Model file for the job. Use its own axes, mm. A direction names the side the tool comes from. Give positions to 0.01 mm unless a question says otherwise; leave off trailing zeros. Loops run counter-clockwise (first coordinate to the right, second up) from the corner with the lowest first, then second, coordinate; pieces in that order, holes last. Notation, with made-up numbers: M 19.25,88 L 40.25,88 A28 cw 40.25,117 Z; hole C -24.5,47 d1. An arc over 180 degrees is marked long. Answer in a Markdown table with one row per item.
Autodesk Inventor part; units mm, degrees
ref_plane "Work Plane1" through (-25.4, 0, 31.75) normal (0, 0, 1) x (1, 0, 0)
ref_plane "YZ Plane" through (0, 0, 0) normal (1, 0, 0) x (0, 1, 0)
ref_plane "XZ Plane" through (0, 0, 0) normal (0, 1, 0) x (-1, 0, 0)
sketch "Sketch1" plane through (0, 0, 0) normal (0, 1, 0) x (-1, 0, 0)
  line L0 (-25.4, 57.15) -> (25.4, 57.15)
  line L1 (25.4, 57.15) -> (25.4, -57.15)
  line L2 (25.4, -57.15) -> (-25.4, -57.15)
  line L3 (-25.4, -57.15) -> (-25.4, 57.15)
  line L4 (-25.4, 57.15) -> (25.4, -57.15) construction
  line L5 (25.4, 57.15) -> (-25.4, -57.15) construction
  point P0 (0, 0)
  dimension "d0" = 50.8
  dimension "d1" = 114.3
extrude "Extrusion1" add sketch "Sketch1" along normal blind 15.875
ref_plane "Work Plane1" through (-25.4, 0, 31.75) normal (0, 0, 1) x (1, 0, 0)
sketch "Sketch2" plane through (-25.4, 0, 31.75) normal (0, 0, 1) x (1, 0, 0)
  line L0 (50.8, 0) -> (0, 0) construction
  line L1 (50.8, 0) -> (50.8, 15.875) construction
  line L2 (0, 15.875) -> (50.8, 15.875) construction
  line L3 (0, 0) -> (0, 15.875) construction
  line L4 (0, 15.875) -> (50.8, 15.875) construction
  line L5 (25.4, 15.875) -> (25.4, 0) construction
  line L6 (50.8, 0) -> (0, 0) construction
  line L7 (6.35, 15.875) -> (6.35, 0) construction
  circle A0 centre (25.4, 16.891) radius 5.08 construction
  line L8 (12.7, 15.875) -> (12.7, 12.7)
  line L9 (12.7, 12.7) -> (9.525, 10.8669)
  line L10 (9.525, 10.8669) -> (9.525, 7.9375)
  line L11 (9.525, 7.9375) -> (19.05, 7.9375)
  line L12 (19.05, 7.9375) -> (19.05, 3.175)
  line L13 (19.05, 3.175) -> (25.4, 3.175)
  line L14 (12.7, 15.875) -> (25.4, 15.875)
  line L15 (25.4, 15.875) -> (25.4, 3.175)
  line L16 (19.05, 7.9375) -> (25.4, 7.9375)
  line L17 (20.6375, 7.9375) -> (20.6375, 7.2665)
  line L18 (20.6375, 7.2665) -> (22.225, 6.35)
  line L19 (22.225, 6.35) -> (22.225, 3.175)
  point P0 (22.225, 4.7625)
  point P1 (19.05, 5.5562)
  dimension "d20" = 6.35
  dimension "d21" = 10.16
  dimension "d22" = 6.35
  dimension "d23" = 4.7625
  dimension "d24" = 3.175
  dimension "d25" = 3.175
  dimension "d26" = 30
  dimension "d27" = 3.175
  dimension "d28" = 3.175
  dimension "d29" = 1.016
  dimension "d45" = 1.5875
  dimension "d46" = 3.175
  dimension "d48" = 3.175
  dimension "d50" = 30
extrude "Extrusion2" cut sketch "Sketch2" against normal through all
extrude "Extrusion3" cut sketch "Sketch2" along normal through all contours L14 L15 L16 L11 L10 L9 L8 | L17 L18 L19 L13 L12 L16
sketch "Sketch7" plane through (-6.35, 3.175, -57.15) normal (0, 1, 0) x (1, 0, 0)
  line L0 (0, -114.3) -> (0, 0) construction
  line L1 (6.35, -114.3) -> (1.5875, -114.3) construction
  line L2 (6.35, -88.9) -> (6.35, -114.3) construction
  line L3 (1.5875, -88.9) -> (6.35, -88.9) construction
  line L4 (1.5875, -88.9) -> (1.5875, -114.3) construction
  line L5 (0, -87.63) -> (1.5875, -86.0425)
  line L6 (1.5875, -86.0425) -> (1.5875, 0)
  line L7 (-19.05, 0) -> (31.75, 0)
  line L8 (0, 0) -> (1.5875, 0)
  line L9 (0, 0) -> (0, -87.63)
  point P0 (6.35, -57.15)
  dimension "d63" = 135
  dimension "d64" = 1.5875
  dimension "d65" = 1.27
extrude "Extrusion6" add sketch "Sketch7" along normal up to surface (4.7625 mm away)
chamfer "Chamfer2" distance 0.762 angle 45 2 edges at (-4.7625, 7.602, 31.75) (-3.175, 4.7625, 57.15)
sketch "Sketch8" plane through (0, 15.875, 0) normal (0, 1, 0) x (1, 0, 0)
  circle A0 centre (-20.32, 26.67) radius 2.5797 construction
  line L0 (-12.7, 57.15) -> (-25.4, 57.15) construction
  line L1 (-25.4, 57.15) -> (-25.4, -57.15) construction
  line L2 (-15.875, -57.15) -> (-15.875, 57.15) construction
  line L3 (-25.4, -57.15) -> (25.4, -57.15)
  line L4 (-25.4, 22.86) -> (-19.05, 16.51)
  line L5 (-19.05, 16.51) -> (-19.05, -41.91)
  line L6 (-19.05, -41.91) -> (-25.4, -48.26)
  line L7 (-25.4, 22.86) -> (-25.4, -48.26)
  line L8 (-25.4, -57.15) -> (-25.4, 57.15) construction
  line L9 (-25.4, 30.48) -> (-19.05, 36.83)
  line L10 (-19.05, 36.83) -> (-19.05, 57.15)
  line L11 (-25.4, 30.48) -> (-25.4, 22.86) construction
  line L12 (-25.4, 30.48) -> (-25.4, 57.15)
  line L13 (-25.4, 57.15) -> (-19.05, 57.15)
  point P0 (0, 0)
  point P1 (-20.32, -52.07)
  point P2 (-12.7, -57.15)
  point P3 (-25.4, 26.67)
  dimension "d71" = 5.1594
  dimension "d72" = 30.48
  dimension "d73" = 5.08
  dimension "d75" = 135
  dimension "d76" = 135
  dimension "d77" = 3.175
  dimension "d89" = 34.29
  dimension "d91" = 5.08
  dimension "d92" = 8.89
hole "Hole2" at (-20.32, 15.875, -26.67) at (-20.32, 15.875, 52.07) direction (0, -1, 0) diameter 5.1562 end through all
extrude "Extrusion7" cut sketch "Sketch8" against normal through all
mirror "Mirror1" about plane through (0, 15.875, 31.75) normal (-1, 0, 0) of "Extrusion2", "Extrusion3", "Extrusion7", "Hole2", "Chamfer2", "Extrusion6"
sketch "Sketch9" plane through (0, 0, 0) normal (0, -1, 0) x (1, 0, 0)
  line L0 (19.05, -57.15) -> (19.05, -36.83)
  line L1 (19.05, -57.15) -> (12.7, -57.15)
  line L2 (-19.05, -57.15) -> (-19.05, -36.83)
  line L3 (19.05, -57.15) -> (-19.05, -57.15)
  line L4 (-19.05, -57.15) -> (-19.05, -40.64)
  line L5 (-19.05, -40.64) -> (19.05, -40.64)
  line L6 (19.05, -40.64) -> (19.05, -57.15)
  point P0 (0, 0)
  dimension "d93" = 16.51
extrude "Extrusion8" cut sketch "Sketch9" against normal through all
equation "\"d76\" = d75"
properties part number "Holder_Mount" material "ABS Plastic"
Q1. Saw through at C-C (y = 1.75). Give the cut face in (x, z), and give its area (3 significant figures).
Reported:
| item | result |
|---|---|
| outline | M -25.4,-30.48 L -19.05,-36.83 L -19.05,-40.64 L 19.05,-40.64 L 19.05,-36.83 L 25.4,-30.48 L 25.4,-22.86 L 19.05,-16.51 L 19.05,41.91 L 25.4,48.26 L 25.4,57.15 L -25.4,57.15 L -25.4,48.26 L -19.05,41.91 L -19.05,-16.51 L -25.4,-22.86 Z; hole C -20.32,-26.67 d5.16; hole C -20.32,52.07 d5.16; hole C 20.32,-26.67 d5.16; hole C 20.32,52.07 d5.16 |
| area | 3,970 mm² |
Q2. Saw through at B-B (x = -20.32). Give the cut face in (y, z) (3 decimals), and give its area (3 significant figures).
Reported:
| item | result |
|---|---|
| outline | M 0,-35.56 L 15.875,-35.56 L 15.875,-29.248 L 0,-29.248 Z; M 0,-24.092 L 15.875,-24.092 L 15.875,-17.78 L 0,-17.78 Z; M 0,43.18 L 15.875,43.18 L 15.875,49.492 L 0,49.492 Z; M 0,54.648 L 15.875,54.648 L 15.875,57.15 L 0,57.15 Z |
| area | 340 mm² |
Q3. 3-axis set-ups, long thin cutter, end or side, ignore diameter. For faces 4 (the face through (-15.875, 9, 8)), 5 (the face through (-19.05, 8, -39)), 6 (the face through (-22.27, 8.05, -19.73)): which of +Z, -Z, +X, -X, +Y, -Y reach the whole face in a straight line?
Reported:
| item | result |
|---|---|
| face 4 | +Z, -Z |
| face 5 | -Z, -X, +Y, -Y |
| face 6 | -X, +Y, -Y |
Q4. Saw through at A-A (z = -26.67). Give the cut face in (x, y) (1 decimal).
Reported:
| item | result |
|---|---|
| outline | M -25.4,0 L -22.9,0 L -22.9,15.9 L -25.4,15.9 Z; M -17.7,0 L 17.7,0 L 17.7,15.9 L 12.7,15.9 L 12.7,12.7 L 15.9,10.9 L 15.9,7.9 L 4.8,7.9 L 4.8,3.2 L -4.8,3.2 L -4.8,7.9 L -15.9,7.9 L -15.9,10.9 L -12.7,12.7 L -12.7,15.9 L -17.7,15.9 Z; M 22.9,0 L 25.4,0 L 25.4,15.9 L 22.9,15.9 Z |
Q5. Probe probe 1 along X at (y, z) = (3.5, -26.67); probe 2 along X at (y, z) = (7.75, 34); probe 3 along X at (y, z) = (5.5, 52.07) (3 decimals). List the from-to ranges inside material, lowest first.
Reported:
| item | result |
|---|---|
| probe 1 | -25.4 to -22.9, -17.74 to -4.76, 4.76 to 17.74, 22.9 to 25.4 |
| probe 2 | -19.05 to -6.35, -4.76 to 4.76, 6.35 to 19.05 |
| probe 3 | -25.4 to -22.898, -17.742 to -6.35, -3.175 to 3.175, 6.35 to 17.742, 22.898 to 25.4 |
Q6. Drop flat-ended pins along their axis: pin 1 (2.5 mm diameter, centred on y = 4.5, z = 38.5, fed in from +X); pin 2 (5 mm diameter, centred on x = 2, z = 46.5, fed in from +Y); pin 3 (3 mm diameter, centred on y = 9.5, z = -38.5, fed in from -X). Give the stop position or say it passes through.
Reported:
| item | result |
|---|---|
| pin 1 | x = 19.05 |
| pin 2 | y = 7.94 |
| pin 3 | x = -19.05 |
Q7. Mould opens along Z. For faces 1 (the face through (-17.803, 7.826, 51.511)), 2 (the face through (4.09, 6.88, 44.27)), 3 (the face through (0, 6, 31.75)) say: released by +Z, released by -Z, zero draft, split by the parting line, or undercut.
Reported:
| item | result |
|---|---|
| face 1 | undercut |
| face 2 | zero draft |
| face 3 | released by -Z |
